Part model, mm, in its own coordinate system. A direction names the side the tool comes from. Give positions to 0.01 mm unless a question says otherwise; leave off trailing zeros. Write each loop counter-clockwise with the first axis right and the second up, starting at its lowest first coordinate (ties: lowest second). Pieces come first, ordered by that corner, then holes. Notation, with made-up numbers: (-6.75, 0.25) - (48.25, 0.25) arc R29 cw to (48.25, 37.25) - close; hole circle Ø2 at (33.5, -2). An arc over 180 degrees is marked (long way). Answer as a JSON object with one key per item and string values. Group by question number.
```python
from build123d import *

# Parameters (mm, degrees)
F0_W     = 100
F0_H     = 100
F1_DEPTH = 100
F2_T     = -5
F3_R     = 20


with BuildPart() as f1:
    # F0 (on Top) → F1 (new body)
    with BuildSketch(Plane.XY):
        with Locations((50, 50)):
            Rectangle(F0_W, F0_H)
    extrude(amount=F1_DEPTH)

    # F2
    f2_openings = [f1.faces().sort_by_distance(p)[0] for p in [
        (50, 0, 50),
    ]]
    offset(amount=F2_T, openings=f2_openings)

    # F3
    f3_edges = [f1.edges().sort_by_distance(p)[0] for p in [
        (95, 47.5, 95),
        (95, 47.5, 5),
        (5, 47.5, 5),
        (5, 47.5, 95),
    ]]
    fillet(f3_edges, radius=F3_R)


solid = f1.part
```
1) Two-plate mould, pull along Z, no slides. Class faces 1 (the flat face through (49, 95, 49)), 2 (the flat face through (0, 49, 49)), 3 (the flat face through (49, 51, 100)): +Z half, -Z half, draft (parallel to the pull), parting line (faces both ways), or undercut.
2) Drop a flat-ended pin along its axis: P1, Ø12, axis at x = 48.5, z = 44, coming from the -Y side. Give the stop position or say it passes through.
3) Drill centre lines: line 1 along X through (y, z) = (64.5, 41); line 2 along Y through (x, z) = (57.5, 66). Where is each one in solid material? Low to high. Write a range as from..to.
4) Which spindle directions (+Z, -Z, +X, -X, +Y, -Y) get a long thin tool onto all of the face, cutting with end or side? Do faces 4 (the flat face through (100, 49, 49)), 5 (the cylindrical face through (89.297, 48.165, 11.014)). Say none if no direction does.
5) Saw through at B-B (x = 32). List the corners of the cut face in (y, z), and give its area (3 significant figures).
6) Saw through at C-C (z = 91). List the corners of the cut face in (x, y).
7) Saw through at A-A (y = 47). List the corners of the cut face in (x, z).
Checks:
{
 "1": {"face 1": "undercut", "face 2": "draft", "face 3": "+Z half"},
 "2": {"P1": "y = 95"},
 "3": {"line 1": "0..5, 95..100", "line 2": "95..100"},
 "4": {"face 4": "+Z, -Z, +X, +Y, -Y", "face 5": "-Y"},
 "5": {"outline": "(0, 0) - (100, 0) - (100, 100) - (0, 100) - (0, 95) - (95, 95) - (95, 5) - (0, 5) - close", "area": "1,450 mm2"},
 "6": {"outline": "(0, 0) - (13, 0) - (13, 95) - (87, 95) - (87, 0) - (100, 0) - (100, 100) - (0, 100) - close"},
 "7": {"outline": "(0, 0) - (100, 0) - (100, 100) - (0, 100) - close; hole (5, 25) arc R20 ccw to (25, 5) - (75, 5) arc R20 ccw to (95, 25) - (95, 75) arc R20 ccw to (75, 95) - (25, 95) arc R20 ccw to (5, 75) - close"}
}
